```python
from build123d import *

# Parameters (mm, degrees)
SKETCH077_W     = 13
SKETCH077_H     = 39
SKETCH077_R     = 1.75
PAD053_DEPTH    = 4
SKETCH082_W     = 13
SKETCH082_H     = 4
PAD054_DEPTH    = 53
SKETCH083_W     = 13
SKETCH083_H     = 39
SKETCH083_R     = 1.75
PAD055_DEPTH    = 4
SKETCH084_R     = 1.75
POCKET017_DEPTH = 4
SKETCH085_R     = 1.75
POCKET018_DEPTH = 4


with BuildPart() as part:
    # Sketch077 → Pad053 (new body)
    with BuildSketch(Plane.XZ):
        with Locations((0, -19.7)):
            Rectangle(SKETCH077_W, SKETCH077_H)
        with Locations((0, -10.7)):
            Circle(SKETCH077_R, mode=Mode.SUBTRACT)
        with Locations((0, -28.7)):
            Circle(SKETCH077_R, mode=Mode.SUBTRACT)
    extrude(amount=PAD053_DEPTH)

    # Sketch082 (on Face7 of Pad053) → Pad054 (join)
    with BuildSketch(Plane(origin=(0, 0, 0), x_dir=(1, 0, 0), z_dir=(0, 1, 0))):
        with Locations((0, 37.2)):
            Rectangle(SKETCH082_W, SKETCH082_H)
        with Locations((0, 2.2)):
            Rectangle(SKETCH082_W, SKETCH082_H)
    extrude(amount=PAD054_DEPTH)

    # Sketch083 (on Face12 of Pad054) → Pad055 (join)
    with BuildSketch(Plane(origin=(0, 53, 0), x_dir=(1, 0, 0), z_dir=(0, 1, 0))):
        with Locations((0, 19.7)):
            Rectangle(SKETCH083_W, SKETCH083_H)
        with Locations((0, 28.7)):
            Circle(SKETCH083_R, mode=Mode.SUBTRACT)
        with Locations((0, 10.7)):
            Circle(SKETCH083_R, mode=Mode.SUBTRACT)
    extrude(amount=PAD055_DEPTH)

    # Sketch084 (on Face18 of Pad055) → Pocket017 (cut)
    with BuildSketch(Plane(origin=(0, 0, -4.2), x_dir=(1, 0, 0), z_dir=(0, 0, -1))):
        with Locations((0, -6.5)):
            Circle(SKETCH084_R)
        with Locations((0, -46.5)):
            Circle(SKETCH084_R)
    extrude(amount=-POCKET017_DEPTH, mode=Mode.SUBTRACT)

    # Sketch085 (on Face15 of Pad054) → Pocket018 (cut)
    with BuildSketch(Plane(origin=(0, 0, -39.2), x_dir=(1, 0, 0), z_dir=(0, 0, -1))):
        with Locations((0, -24.5)):
            Circle(SKETCH085_R)
    extrude(amount=-POCKET018_DEPTH, mode=Mode.SUBTRACT)


with BuildPart() as part_1:
    # Body018 placement: moved
    add(part.part.moved(Location((0, -26.5, 0))))


solid = part_1.part
```
Read the model definition and answer for the solid it produces. Units are mm, in the model's axes. A direction names the side the tool comes from. Give positions to 0.01 mm unless a question says otherwise; leave off trailing zeros. Loops run counter-clockwise (first coordinate to the right, second up) from the corner with the lowest first, then second, coordinate; pieces in that order, holes last.
Item 1: The part is cut by section B-B (y = 8). Write down the section's boundary in (x, z).
Item 2: Find the intervals of material crossed by line 1 along Z through (x, y) = (0, 29); line 2 along Y through (x, z) = (0, -3.1); line 3 along Z through (x, y) = (-4.25, 8), in increasing order.
Item 3: The part is cut by section A-A (z = -23.5). Write down the section's boundary in (x, y).
Item 4: The mould has two halves that part along X. Classify faces 1 (the flat face through (0, -30.5, -19)), 2 (the flat face through (6.5, 0, -37)), 3 (the cylindrical face through (-0.228, -21.735, -2.228)), 4 (the cylindrical face through (0.81, -0.45, -37.23)): released by +X, released by -X, zero draft, split by the parting line, or undercut.
Item 5: The part is cut by section C-C (z = -28.7). Write down the section's boundary in (x, y).
Item 6: The part is cut by section D-D (y = 20). Write down the section's boundary in (x, z), and give its area (3 significant figures).
Item 7: Each of these flat-tipped pins is pushed along its axis until it touches: pin 1 Ø4.5 at (x, z) = (0, -10.7) entering from -Y; pin 2 Ø2 at (x, y) = (0, -2) entering from -Z. Where does it stop, or does it pass through?
Item 8: For faces 5 (the flat face through (-2, 0, -39.2)), 6 (the flat face through (0, -26.5, -19)), 7 (the cylindrical face through (-0.228, 18.265, -2.228)), determine the directions among +Z, -Z, +X, -X, +Y, -Y from which every point of the face is accessible in a straight line to the end or side of a thin tool.
Taken from the geometry:
1. outline: (-6.5, -39.2) - (6.5, -39.2) - (6.5, -35.2) - (-6.5, -35.2) - close; (-6.5, -4.2) - (6.5, -4.2) - (6.5, -0.2) - (-6.5, -0.2) - close
2. line 1: z = -39.2 to -30.45, -26.95 to -12.45, -8.95 to -0.2
2. line 2: y = -30.5 to -21.75, -18.25 to 18.25, 21.75 to 30.5
2. line 3: z = -39.2 to -35.2, -4.2 to -0.2
3. outline: (-6.5, -30.5) - (6.5, -30.5) - (6.5, -26.5) - (-6.5, -26.5) - close; (-6.5, 26.5) - (6.5, 26.5) - (6.5, 30.5) - (-6.5, 30.5) - close
4. face 1: zero draft
4. face 2: released by +X
4. face 3: undercut
4. face 4: undercut
5. outline: (-6.5, -30.5) - (-1.75, -30.5) - (-1.75, -26.5) - (-6.5, -26.5) - close; (-6.5, 26.5) - (-1.75, 26.5) - (-1.75, 30.5) - (-6.5, 30.5) - close; (1.75, -30.5) - (6.5, -30.5) - (6.5, -26.5) - (1.75, -26.5) - close; (1.75, 26.5) - (6.5, 26.5) - (6.5, 30.5) - (1.75, 30.5) - close
6. outline: (-6.5, -39.2) - (6.5, -39.2) - (6.5, -35.2) - (-6.5, -35.2) - close; (-6.5, -4.2) - (-1.75, -4.2) - (-1.75, -0.2) - (-6.5, -0.2) - close; (1.75, -4.2) - (6.5, -4.2) - (6.5, -0.2) - (1.75, -0.2) - close
6. area: 90.0 mm2
7. pin 1: stops at y = -30.5
7. pin 2: stops at z = -4.2
8. face 5: -Z, +X, -X, +Y, -Y
8. face 6: +X, -X
8. face 7: +Z
